Geometry check sheet. Reference: the model listing, model coordinates, mm. A direction names the side the tool comes from. Round coordinates to 2 decimals unless told otherwise and drop trailing zeros. Write each loop counter-clockwise with the first axis right and the second up, starting at its lowest first coordinate (ties: lowest second). Pieces come first, ordered by that corner, then holes. Notation, with made-up numbers: (72.5, 0) -> (84.5, 0) arc R31 cw to (84.5, 26) -> close; hole circle Ø5 at (54, 74). An arc over 180 degrees is marked (long way). One line per question, with ' | ' between items.
```python
from build123d import *

# Parameters (mm, degrees)
SKETCH1_W           = 50
SKETCH1_H           = 10
BOSS_EXTRUDE1_DEPTH = 1.5
SKETCH3_W           = 5
SKETCH3_H           = 1.5
CUT_EXTRUDE1_DEPTH  = 2
SKETCH2_R           = 1
CUT_EXTRUDE2_DEPTH  = 2


with BuildPart() as part:
    # Sketch1 → Boss-Extrude1 (new body)
    with BuildSketch(Plane(origin=(0, 0, 0), x_dir=(1, 0, 0), z_dir=(0, 1, 0))):
        with Locations((15.170187286, 0.880693734)):
            Rectangle(SKETCH1_W, SKETCH1_H)
    extrude(amount=BOSS_EXTRUDE1_DEPTH)

    # Sketch3 → Cut-Extrude1 (cut)
    with BuildSketch(Plane(origin=(0, 1.5, 0), x_dir=(1, 0, 0), z_dir=(0, 1, 0))):
        with Locations((10.170187286, 2.630693734)):
            Rectangle(SKETCH3_W, SKETCH3_H)
        with Locations((20.170187286, 2.630693734)):
            Rectangle(SKETCH3_W, SKETCH3_H)
        with Locations((20.170187286, -0.869306266)):
            Rectangle(SKETCH3_W, SKETCH3_H)
        with Locations((10.170187286, -0.869306266)):
            Rectangle(SKETCH3_W, SKETCH3_H)
    extrude(amount=-CUT_EXTRUDE1_DEPTH, mode=Mode.SUBTRACT)

    # Sketch2 → Cut-Extrude2 (cut)
    with BuildSketch(Plane(origin=(0, 1.5, 0), x_dir=(1, 0, 0), z_dir=(0, 1, 0))):
        with Locations((15.170187286, 0.880693734)):
            Circle(SKETCH2_R)
    extrude(amount=-CUT_EXTRUDE2_DEPTH, mode=Mode.SUBTRACT)


solid = part.part
```
(1) Material ranges on line 1 (X direction, y = 0.15, z = 0.5); line 2 (Z direction, x = 12, y = 1.25); line 3 (X direction, y = 0.6, z = -1), recorded low to high.
Resolved:
line 1: x = -9.83 to 7.67, 12.67 to 17.67, 22.67 to 40.17 | line 2: z = -5.88 to -3.38, -1.88 to 0.12, 1.62 to 4.12 | line 3: x = -9.83 to 14.18, 16.16 to 40.17
(2) Access from +Z, -Z, +X, -X, +Y, -Y to the whole of each face (thin tool, end or side, straight path). Record for faces 4 (the flat face through (17.67, 1, -3)), 5 (the flat face through (40.17, 1, -1)).
Resolved:
face 4: +Y, -Y | face 5: +Z, -Z, +X, +Y, -Y
(3) Sectioned sample at A-A on x = 10.5. Record the cut outline in (y, z).
Resolved:
outline: (0, -5.88) -> (1.5, -5.88) -> (1.5, -3.38) -> (0, -3.38) -> close; (0, -1.88) -> (1.5, -1.88) -> (1.5, 0.12) -> (0, 0.12) -> close; (0, 1.62) -> (1.5, 1.62) -> (1.5, 4.12) -> (0, 4.12) -> close
(4) Draft check along Z on faces 1 (the flat face through (14.8, 0, -2.1)), 2 (the flat face through (15, 1, 4.119)), 3 (the flat face through (20, 1, -3.381)). Enter one of: +Z half, -Z half, draft (parallel to the pull), parting line (faces both ways), or undercut.
Resolved:
face 1: draft | face 2: +Z half | face 3: undercut
(5) Sectioned sample at B-B on y = 0.95. Record the cut outline in (x, z), then the cut area to 3 significant figures.
Resolved:
outline: (-9.83, -5.88) -> (40.17, -5.88) -> (40.17, 4.12) -> (-9.83, 4.12) -> close; hole (7.67, -3.38) -> (12.67, -3.38) -> (12.67, -1.88) -> (7.67, -1.88) -> close; hole (7.67, 0.12) -> (12.67, 0.12) -> (12.67, 1.62) -> (7.67, 1.62) -> close; hole circle Ø2 at (15.17, -0.88); hole (17.67, -3.38) -> (22.67, -3.38) -> (22.67, -1.88) -> (17.67, -1.88) -> close; hole (17.67, 0.12) -> (22.67, 0.12) -> (22.67, 1.62) -> (17.67, 1.62) -> close | area: 467 mm2
